Geometry check sheet. Reference: the model listing, model coordinates, mm. Give positions to 0.01 mm unless a question says otherwise; leave off trailing zeros. Order: outer loops, then holes, each group sorted by start corner. A loop starts at its lowest first (then second) coordinate and runs counter-clockwise, first axis right, second up.
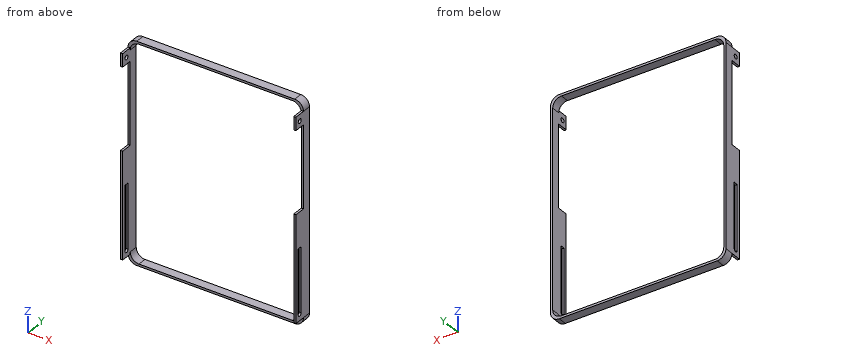
from build123d import *

# Parameters (mm, degrees)
BOSS_EXTRUDE2_DEPTH     = 20
CUT_EXTRUDE1_DEPTH      = 20
SKETCH7_W               = 242.556539121
SKETCH7_H               = 25
BOSS_EXTRUDE3_DEPTH     = 5
SKETCH8_W               = 242.556539121
SKETCH8_H               = 25
BOSS_EXTRUDE4_DEPTH     = 5
CUT_EXTRUDE2_DEPTH      = 473.361090692
CUT_EXTRUDE2_DEPTH_BACK = 473.361090692
SKETCH11_W              = 30
SKETCH11_H              = 25
BOSS_EXTRUDE5_DEPTH     = 5
SKETCH13_W              = 30
SKETCH13_H              = 25
BOSS_EXTRUDE6_DEPTH     = 5
SKETCH14_R              = 5
CUT_EXTRUDE3_DEPTH      = 473.361090692
BOSS_EXTRUDE7_DEPTH     = 5
BOSS_EXTRUDE8_START     = -5
BOSS_EXTRUDE8_DEPTH     = 5


with BuildPart() as part:
    # Sketch5 → Boss-Extrude2 (new body)
    with BuildSketch(Plane(origin=(0, 0, 0), x_dir=(1, 0, 0), z_dir=(0, 1, 0))):
        with BuildLine():
            Line((-180, 250), (180, 250))
            ThreePointArc((180, 250), (194.142135624, 244.142135624), (200, 230))
            Line((200, 230), (200, -230))
            ThreePointArc((200, -230), (194.142135624, -244.142135624), (180, -250))
            Line((180, -250), (-180, -250))
            ThreePointArc((-180, -250), (-194.142135624, -244.142135624), (-200, -230))
            Line((-200, -230), (-200, 230))
            ThreePointArc((-200, 230), (-194.142135624, 244.142135624), (-180, 250))
        make_face()
    extrude(amount=BOSS_EXTRUDE2_DEPTH)

    # Sketch6 → Cut-Extrude1 (cut)
    with BuildSketch(Plane(origin=(0, 20, 0), x_dir=(1, 0, 0), z_dir=(0, 1, 0))):
        with BuildLine():
            Line((-175, -245), (175, -245))
            ThreePointArc((175, -245), (189.142135624, -239.142135624), (195, -225))
            Line((195, -225), (195, 225))
            ThreePointArc((195, 225), (189.142135624, 239.142135624), (175, 245))
            Line((175, 245), (-175, 245))
            ThreePointArc((-175, 245), (-189.142135624, 239.142135624), (-195, 225))
            Line((-195, 225), (-195, -225))
            ThreePointArc((-195, -225), (-189.142135624, -239.142135624), (-175, -245))
        make_face()
    extrude(amount=-CUT_EXTRUDE1_DEPTH, mode=Mode.SUBTRACT)

    # Sketch7 → Boss-Extrude3 (add)
    with BuildSketch(Plane(origin=(200, 0, 0), x_dir=(0, 0, -1), z_dir=(1, 0, 0))):
        with Locations((108.72173044, -12.5)):
            Rectangle(SKETCH7_W, SKETCH7_H)
    extrude(amount=-BOSS_EXTRUDE3_DEPTH)

    # Sketch8 → Boss-Extrude4 (add)
    with BuildSketch(Plane.ZY.offset(200)):
        with Locations((-108.72173044, -12.5)):
            Rectangle(SKETCH8_W, SKETCH8_H)
    extrude(amount=-BOSS_EXTRUDE4_DEPTH)

    # Sketch10 → Cut-Extrude2 (cut, two sides: drawn at the far end of the back side and taken through both)
    with BuildSketch(Plane(origin=(200, 0, 0), x_dir=(0, 0, -1), z_dir=(1, 0, 0)).offset(-CUT_EXTRUDE2_DEPTH_BACK)):
        with BuildLine():
            Line((214.975112076, -7.5), (2.443460879, -7.5))
            ThreePointArc((2.443460879, -7.5), (-2.556539121, -12.5), (2.443460879, -17.5))
            Line((2.443460879, -17.5), (214.975112076, -17.5))
            ThreePointArc((214.975112076, -17.5), (219.975112076, -12.5), (214.975112076, -7.5))
        make_face()
    extrude(amount=CUT_EXTRUDE2_DEPTH + CUT_EXTRUDE2_DEPTH_BACK, mode=Mode.SUBTRACT)

    # Sketch11 → Boss-Extrude5 (add)
    with BuildSketch(Plane(origin=(200, 0, 0), x_dir=(0, 0, -1), z_dir=(1, 0, 0))):
        with Locations((-215, -12.5)):
            Rectangle(SKETCH11_W, SKETCH11_H)
    extrude(amount=-BOSS_EXTRUDE5_DEPTH)

    # Sketch13 → Boss-Extrude6 (add)
    with BuildSketch(Plane.ZY.offset(200)):
        with Locations((215, -12.5)):
            Rectangle(SKETCH13_W, SKETCH13_H)
    extrude(amount=-BOSS_EXTRUDE6_DEPTH)

    # Sketch14 → Cut-Extrude3 (cut, through all)
    with BuildSketch(Plane.ZY.offset(200)):
        with Locations((215, -12.5)):
            Circle(SKETCH14_R)
    extrude(amount=-CUT_EXTRUDE3_DEPTH, mode=Mode.SUBTRACT)

    # Sketch16 → Boss-Extrude7 (add)
    with BuildSketch(Plane.ZY.offset(200)):
        with BuildLine():
            Line((-67.443460879, -17.5), (-2.443460879, -17.5))
            ThreePointArc((-2.443460879, -17.5), (2.556539121, -12.5), (-2.443460879, -7.5))
            Line((-2.443460879, -7.5), (-67.443460879, -7.5))
            Line((-67.443460879, -7.5), (-67.443460879, -17.5))
        make_face()
    extrude(amount=-BOSS_EXTRUDE7_DEPTH)

    # Sketch17 → Boss-Extrude8 (add)
    with BuildSketch(Plane(origin=(200, 0, 0), x_dir=(0, 0, -1), z_dir=(1, 0, 0)).offset(BOSS_EXTRUDE8_START)):
        with BuildLine():
            Line((67.443460879, -17.5), (67.443460879, -7.5))
            Line((67.443460879, -7.5), (2.443460879, -7.5))
            ThreePointArc((2.443460879, -7.5), (-2.556539121, -12.5), (2.443460879, -17.5))
            Line((2.443460879, -17.5), (67.443460879, -17.5))
        make_face()
    extrude(amount=BOSS_EXTRUDE8_DEPTH)


solid = part.part
Item 1: Scan lines: L1, parallel to Z at x = -197, y = -12; L2, parallel to Y at x = 198.8, z = 215; L3, parallel to X at y = -3, z = -174. Record each from-to range of solid material in increasing order.
Reported:
L1: z = -230 to -219.95, -67.44 to 12.56, 200 to 210.03, 219.97 to 230
L2: y = -25 to -17.5, -7.5 to 20
L3: x = -200 to -195, 195 to 200
Item 2: Sectioned sample at B-B (x = 60). Enter the section's corners in (y, z), and give its area (3 significant figures).
Reported:
outline: (0, -250) - (20, -250) - (20, -245) - (0, -245) - close; (0, 245) - (20, 245) - (20, 250) - (0, 250) - close
area: 200 mm2
Item 3: Sectioned sample at D-D (y = 13). Enter the section's corners in (x, z), and give its area (3 significant figures).
Reported:
outline: (-200, -230) arc R20 ccw to (-180, -250) - (180, -250) arc R20 ccw to (200, -230) - (200, 230) arc R20 ccw to (180, 250) - (-180, 250) arc R20 ccw to (-200, 230) - close; hole (-195, -225) arc R20 ccw to (-175, -245) - (175, -245) arc R20 ccw to (195, -225) - (195, 225) arc R20 ccw to (175, 245) - (-175, 245) arc R20 ccw to (-195, 225) - close
area: 8,900 mm2
Item 4: Sectioned sample at C-C (z = 170.5). Enter the section's corners in (x, y), and give its area (3 significant figures).
Reported:
outline: (-200, 0) - (-195, 0) - (-195, 20) - (-200, 20) - close; (195, 0) - (200, 0) - (200, 20) - (195, 20) - close
area: 200 mm2
Item 5: Gauge pin test, flat ends, axial feed: pin 1 (4 mm diameter, centred on x = -197, y = -10.5, fed in from +Z); pin 2 (2.5 mm diameter, centred on x = 198, z = 129, fed in from -Y); pin 3 (5.5 mm diameter, centred on x = 197, y = -12.5, fed in from -Z). Record the tip position at first contact, or that the pin passes through.
Reported:
pin 1: stops at z = 230
pin 2: stops at y = 0
pin 3: stops at z = -230
Item 6: Sectioned sample at A-A (z = -125.5). Enter the section's corners in (x, y), and give its area (3 significant figures).
Reported:
outline: (-200, -25) - (-195, -25) - (-195, -17.5) - (-200, -17.5) - close; (-200, -7.5) - (-195, -7.5) - (-195, 20) - (-200, 20) - close; (195, -25) - (200, -25) - (200, -17.5) - (195, -17.5) - close; (195, -7.5) - (200, -7.5) - (200, 20) - (195, 20) - close
area: 350 mm2
